Could you check a few things on this model? Use its own coordinates, in mm. A direction names the side the tool comes from. Round coordinates to 2 decimals unless told otherwise and drop trailing zeros. Order: outer loops, then holes, each group sorted by start corner. A loop starts at its lowest first (then second) coordinate and runs counter-clockwise, first axis right, second up. Notation, with made-up numbers: (-8, 83.5) - (45, 83.5) arc R33 ccw to (45, 111.5) - close; hole circle Ø3 at (25.5, 65.5). An arc over 180 degrees is marked (long way). Use one line per item in the form item = value.
from build123d import *


with BuildPart() as f1:
    # F0 (on Front) → F1 (revolve)
    with BuildSketch(Plane.XZ):
        with BuildLine():
            Line((-6.2, 6.1), (0, 6.1))
            Line((0, 6.1), (0, 13.9))
            Line((0, 13.9), (-12.2, 13.9))
            ThreePointArc((-12.2, 13.9), (-15.028427, 12.728427), (-16.2, 9.9))
            Line((-16.2, 9.9), (-16.2, 6.1))
            Line((-16.2, 6.1), (-6.2, 6.1))
        make_face()
        with BuildLine():
            Line((-6.2, -6.1), (-6.2, 6.1))
            Line((-6.2, 6.1), (-16.2, 6.1))
            Line((-16.2, 6.1), (-16.2, -4.1))
            ThreePointArc((-16.2, -4.1), (-15.614214, -5.514214), (-14.2, -6.1))
            Line((-14.2, -6.1), (-6.2, -6.1))
        make_face()
    revolve(axis=Axis((0, 0, 10), (0, 0, -1)))


solid = f1.part
Item 1: For faces 1 (the face through (-2.86, -5.5, 0.09)), 2 (the face through (0, 0, 13.9)), which set-ups out of +Z, -Z, +X, -X, +Y, -Y let a thin tool reach every point of the face, with its end or its side?
Found:
face_1 = -Z
face_2 = +Z, +X, -X, +Y, -Y
Item 2: If we mould it in two halves opening along X, with no side actions, what happens to faces 3 (the face through (-6, -3, -6.1)), 4 (the face through (0, 0, 6.1)), 5 (the face through (3.512, -15.815, 2.802))? For each: released by +X, released by -X, zero draft, split by the parting line, or undercut.
Found:
face_3 = zero draft
face_4 = undercut
face_5 = split by the parting line
Item 3: Imagine slicing it at A-A on x = 0. Please give me the cut outline in (y, z), plus the area to 3 significant figures.
Found:
outline = (-16.2, -4.1) arc R2 ccw to (-14.2, -6.1) - (-6.2, -6.1) - (-6.2, 6.1) - (6.2, 6.1) - (6.2, -6.1) - (14.2, -6.1) arc R2 ccw to (16.2, -4.1) - (16.2, 9.9) arc R4 ccw to (12.2, 13.9) - (-12.2, 13.9) arc R4 ccw to (-16.2, 9.9) - close
area = 488 mm2
Item 4: Imagine slicing it at C-C on z = 2. Please give me the cut outline in (x, y), plus the area to 3 significant figures.
Found:
outline = circle Ø32.4 at (0, 0); hole circle Ø12.4 at (0, 0)
area = 704 mm2
Item 5: I need wall thicknesses on L1, parallel to Y at x = 0, z = 3.25; L2, parallel to Z at x = 3, y = 4; L3, parallel to Y at x = 3.5, z = -3.5. Which ranges of each line are inside material? Lowest first, please.
Found:
L1 = -16.2 to -6.2, 6.2 to 16.2
L2 = 6.1 to 13.9
L3 = -15.82 to -5.12, 5.12 to 15.82
Item 6: Imagine slicing it at D-D on z = 12.25. Please give me the cut outline in (x, y), plus the area to 3 significant figures.
Found:
outline = circle Ø30.87 at (0, 0)
area = 749 mm2
Item 7: Will these pins go through, and if not, where does the flat tip stop? P1, Ø6, axis at x = 1.5, y = 0, coming from the -Z side; P2, Ø10, axis at y = 11.5, z = 4, coming from the -X side; P3, Ø2, axis at x = 2, z = 4.5, coming from the -Y side.
Found:
P1 = 6.1
P2 = -14.84
P3 = -16.17
